CAD build for the part. Positions are in the model's coordinates, mm. Round coordinates to 2 decimals unless told otherwise and drop trailing zeros. Loops run counter-clockwise (first coordinate to the right, second up) from the corner with the lowest first, then second, coordinate; pieces in that order, holes last.
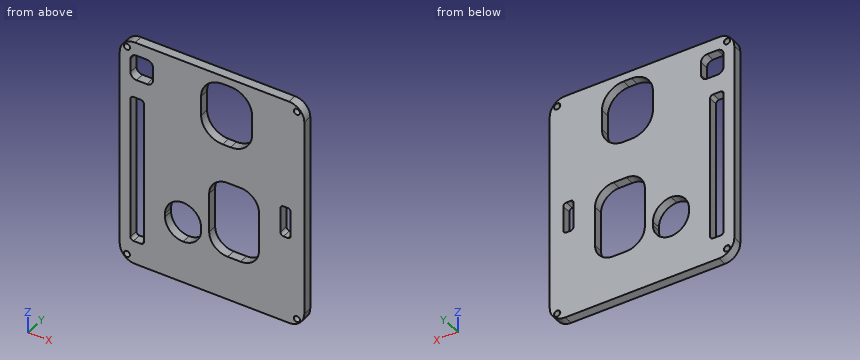
from build123d import *

# Parameters (mm, degrees)
SKIZZE1_W                                = 60
SKIZZE1_H                                = 75
AUFSATZ_LINEAR_AUSTRAGEN1_DEPTH          = 3
VERRUNDUNG1_R                            = 5
F_2_0_2_DURCHMESSER_BOHRUNG1_D           = 2
F_2_0_2_DURCHMESSER_BOHRUNG1_DEPTH       = 20
F_2_0_2_DURCHMESSER_BOHRUNG1_CSINK_D     = 2.05
F_2_0_2_DURCHMESSER_BOHRUNG1_CSINK_ANGLE = 90
F_2_0_2_DURCHMESSER_BOHRUNG1_TIP         = 0.600860619
SKIZZE4_W                                = 25.006881973
SKIZZE4_H                                = 16.195641819
SKIZZE4_W_2                              = 8.317021013
SKIZZE4_H_2                              = 7.361730429
SKIZZE4_W_3                              = 20.485548402
SKIZZE4_H_3                              = 16.578223094
SKIZZE4_W_4                              = 10.159045801
SKIZZE4_H_4                              = 3.349135978
SKIZZE4_W_5                              = 48.785747421
SKIZZE4_H_5                              = 4.403326981
SKIZZE4_W_6                              = 13.233304068
SKIZZE4_H_6                              = 11.709766254
SCHNITT_LINEAR_AUSTRAGEN1_DEPTH          = 5
VERRUNDUNG2_R                            = 6
VERRUNDUNG3_R                            = 1
VERRUNDUNG4_R                            = 7
VERRUNDUNG5_R                            = 2


with BuildPart() as part:
    # Skizze1 → Aufsatz-Linear austragen1 (new body)
    with BuildSketch(Plane(origin=(0, 0, 0), x_dir=(1, 0, 0), z_dir=(0, 1, 0))):
        Rectangle(SKIZZE1_W, SKIZZE1_H)
    extrude(amount=AUFSATZ_LINEAR_AUSTRAGEN1_DEPTH)

    # Verrundung1
    verrundung1_edges = [part.edges().sort_by_distance(p)[0] for p in [
        (30, 1.5, 37.5),
        (-30, 1.5, 37.5),
        (-30, 1.5, -37.5),
        (30, 1.5, -37.5),
    ]]
    fillet(verrundung1_edges, radius=VERRUNDUNG1_R)

    # Ø2.0 (2) Durchmesser Bohrung1
    with Locations(Plane.ZX.offset(3)):
        with Locations((-35.165927774, 27.602462356), (35.054289908, 27.602462356), (35.054289908, -27.658281289), (-35.165927774, -27.658281289)):
            CounterSinkHole(F_2_0_2_DURCHMESSER_BOHRUNG1_D / 2, F_2_0_2_DURCHMESSER_BOHRUNG1_CSINK_D / 2, depth=F_2_0_2_DURCHMESSER_BOHRUNG1_DEPTH, counter_sink_angle=F_2_0_2_DURCHMESSER_BOHRUNG1_CSINK_ANGLE)
            with Locations((0, 0, -(F_2_0_2_DURCHMESSER_BOHRUNG1_DEPTH + F_2_0_2_DURCHMESSER_BOHRUNG1_TIP / 2))):  # 118° drill point
                Cone(0, F_2_0_2_DURCHMESSER_BOHRUNG1_D / 2, F_2_0_2_DURCHMESSER_BOHRUNG1_TIP, mode=Mode.SUBTRACT)

    # Skizze4 → Schnitt-Linear austragen1 (cut)
    with BuildSketch(Plane.ZX.offset(3)):
        with Locations((-10.549778333, 7.176808516)):
            Rectangle(SKIZZE4_W, SKIZZE4_H)
        with Locations((29.109573547, -22.854668692)):
            Rectangle(SKIZZE4_W_2, SKIZZE4_H_2)
        with Locations((24.644058909, 4.744609303)):
            Rectangle(SKIZZE4_W_3, SKIZZE4_H_3)
        with Locations((-3.795687443, 23.91841278)):
            Rectangle(SKIZZE4_W_4, SKIZZE4_H_4)
        with Locations((-5.526074365, -24.333870416)):
            Rectangle(SKIZZE4_W_5, SKIZZE4_H_5)
        with Locations((-17.106394481, -9.399385371)):
            Rectangle(SKIZZE4_W_6, SKIZZE4_H_6)
    extrude(amount=-SCHNITT_LINEAR_AUSTRAGEN1_DEPTH, mode=Mode.SUBTRACT)

    # Verrundung2
    # the kernel refuses this fillet: 6 mm, written as the material it adds along each edge
    with BuildSketch(Plane(origin=(-15.254268498, 3, -23.723046515), x_dir=(1, 0, 0), z_dir=(0, -1, 0)), Plane(origin=(-3.544502244, 3, -23.723046515), x_dir=(0, 0, 1), z_dir=(0, -1, 0)), Plane(origin=(-3.544502244, 3, -10.489742447), x_dir=(-1, 0, 0), z_dir=(0, -1, 0)), Plane(origin=(-0.921012394, 3, -23.053219319), x_dir=(1, 0, 0), z_dir=(0, -1, 0)), Plane(origin=(15.274629425, 3, -23.053219319), x_dir=(0, 0, 1), z_dir=(0, -1, 0)), Plane(origin=(15.274629425, 3, 1.953662654), x_dir=(-1, 0, 0), z_dir=(0, -1, 0))) as verrundung2_piece_1:
        with BuildLine():
            CenterArc((VERRUNDUNG2_R, VERRUNDUNG2_R), VERRUNDUNG2_R, 180, 90)
            Line((0, VERRUNDUNG2_R), (0, 0))
            Line((0, 0), (VERRUNDUNG2_R, 0))
        make_face()
    extrude(amount=3)
    with BuildSketch(Plane(origin=(-15.254268498, 3, -10.489742447), x_dir=(1, 0, 0), z_dir=(0, -1, 0)), Plane(origin=(-0.921012394, 3, 1.953662654), x_dir=(1, 0, 0), z_dir=(0, -1, 0))) as verrundung2_piece_2:
        with BuildLine():
            CenterArc((VERRUNDUNG2_R, -VERRUNDUNG2_R), VERRUNDUNG2_R, 90, 90)
            Line((0, -VERRUNDUNG2_R), (0, 0))
            Line((0, 0), (VERRUNDUNG2_R, 0))
        make_face()
    extrude(amount=3)

    # Verrundung3
    verrundung3_edges = [part.edges().sort_by_distance(p)[0] for p in [
        (-26.535533906, 1.5, -29.918948075),
        (-22.132206925, 1.5, -29.918948075),
        (-22.132206925, 1.5, 18.866799346),
        (-26.535533906, 1.5, 18.866799346),
        (22.243844791, 1.5, -8.875210343),
        (25.592980769, 1.5, -8.875210343),
        (25.592980769, 1.5, 1.283835458),
        (22.243844791, 1.5, 1.283835458),
    ]]
    fillet(verrundung3_edges, radius=VERRUNDUNG3_R)

    # Verrundung4
    verrundung4_edges = [part.edges().sort_by_distance(p)[0] for p in [
        (-3.544502244, 1.5, 14.401284708),
        (13.03372085, 1.5, 14.401284708),
        (13.03372085, 1.5, 34.88683311),
        (-3.544502244, 1.5, 34.88683311),
    ]]
    fillet(verrundung4_edges, radius=VERRUNDUNG4_R)

    # Verrundung5
    verrundung5_edges = [part.edges().sort_by_distance(p)[0] for p in [
        (-26.535533906, 1.5, 24.95106304),
        (-19.173803477, 1.5, 24.95106304),
        (-19.173803477, 1.5, 33.268084053),
        (-26.535533906, 1.5, 33.268084053),
    ]]
    fillet(verrundung5_edges, radius=VERRUNDUNG5_R)


solid = part.part
Item 1: Cut at D-D (z = 20.5). List the corners of the cut face in (x, y).
Verdict:
outline: (-30, 0) - (-3.49, 0) - (-3.49, 3) - (-30, 3) - close; (12.98, 0) - (30, 0) - (30, 3) - (12.98, 3) - close
Item 2: Cut at B-B (z = -15.5). List the corners of the cut face in (x, y).
Verdict:
outline: (-30, 0) - (-26.54, 0) - (-26.54, 3) - (-30, 3) - close; (-22.13, 0) - (-15.17, 0) - (-15.17, 3) - (-22.13, 3) - close; (-3.63, 0) - (-0.92, 0) - (-0.92, 3) - (-3.63, 3) - close; (15.27, 0) - (30, 0) - (30, 3) - (15.27, 3) - close
Item 3: Wall check: L1, parallel to X at y = 0.2, z = -6.5; L2, parallel to Z at x = 5.5, y = 1.6; L3, parallel to Z at x = 1.5, y = 1.15. Give the ranges that are in metal, low to high.
Verdict:
L1: x = -30 to -26.54, -22.13 to -0.92, 15.27 to 22.24, 25.59 to 30
L2: z = -37.5 to -23.05, 1.95 to 14.4, 34.89 to 37.5
L3: z = -37.5 to -21.87, 0.77 to 14.68, 34.61 to 37.5
Item 4: Flat gauge pin, fed straight in: P1, Ø3, axis at x = -27.66, z = 35.05, coming from the +Y side. Where does the tip first touch, or does it go through?
Verdict:
P1: stops at y = 3
Item 5: Cut at C-C (x = 1). List the corners of the cut face in (y, z), plus the area to 3 significant figures.
Verdict:
outline: (0, -37.5) - (3, -37.5) - (3, -21.45) - (0, -21.45) - close; (0, 0.35) - (3, 0.35) - (3, 14.85) - (0, 14.85) - close; (0, 34.44) - (3, 34.44) - (3, 37.5) - (0, 37.5) - close
area: 101 mm2
Item 6: Cut at A-A (x = -8). List the corners of the cut face in (y, z), plus the area to 3 significant figures.
Verdict:
outline: (0, -37.5) - (3, -37.5) - (3, -23.52) - (0, -23.52) - close; (0, -10.69) - (3, -10.69) - (3, 37.5) - (0, 37.5) - close
area: 187 mm2
